The listing builds one solid part. Answer for the finished solid, in the listing's coordinates (mm). A direction names the side the tool comes from. Coordinates: 2 decimals unless noted, no trailing zeros. Order: outer loops, then holes, each group sorted by start corner. A loop starts at its lowest first (then second) coordinate and runs counter-clockwise, first axis right, second up.
Autodesk Inventor part; units mm, degrees
ref_plane "Start Plane" through (0, 0, 25) normal (0, 0, 1) x (1, 0, 0)
ref_plane "End Plane" through (0, 0, 185) normal (0, 0, 1) x (1, 0, 0)
ref_plane "Work Plane4" through (1045, -21, 185) normal (0, 0, 1) x (1, 0, 0)
ref_plane "Start Plane" through (0, 0, 25) normal (0, 0, 1) x (1, 0, 0)
ref_plane "End Plane" through (0, 0, 185) normal (0, 0, 1) x (1, 0, 0)
sketch "Sketch" plane through (0, 0, 0) normal (0, 0, 1) x (1, 0, 0)
  line L0 (-25, -21) -> (-25, 21)
  line L1 (-21, 25) -> (21, 25)
  line L2 (25, 21) -> (25, -21)
  line L3 (21, -25) -> (-21, -25)
  arc A0 (-25, -21) -> (-21, -25) centre (-21, -21) ccw
  arc A1 (25, 21) -> (21, 25) centre (21, 21) ccw
  arc A2 (-21, 25) -> (-25, 21) centre (-21, 21) ccw
  arc A3 (21, -25) -> (25, -21) centre (21, -21) ccw
  arc A4 (-21, 23) -> (-23, 21) centre (-21, 21) ccw
  line L4 (-21, 23) -> (21, 23)
  arc A5 (23, 21) -> (21, 23) centre (21, 21) ccw
  line L5 (23, 21) -> (23, -21)
  arc A6 (21, -23) -> (23, -21) centre (21, -21) ccw
  line L6 (21, -23) -> (-21, -23)
  arc A7 (-23, -21) -> (-21, -23) centre (-21, -21) ccw
  line L7 (-23, -21) -> (-23, 21)
  line L8 (0, 36.1598) -> (0, -36.1598) construction
  line L9 (-36.1598, 0) -> (36.1598, 0) construction
  dimension "d7" = 4
  dimension "d9" = 50
  dimension "d11" = 50
  dimension "d12" = 2
  dimension "d15" = 25
  dimension "d16" = 25
extrude "Body" add sketch "Sketch" along normal up to surface (160 mm away) from surface at 25
sketch "Sketch3" plane through (0, 0, 0) normal (0, 0, 1) x (1, 0, 0)
  line L0 (0, 0) -> (10, 0)
ref_plane "Work Plane3" through (0, 0, 0) normal (0, -1, 0) x (1, 0, 0)
sketch "Sketch4" plane through (0, 0, 0) normal (0, -1, 0) x (1, 0, 0)
  line L0 (-2, 25) -> (12, 25)
  line L1 (-2, 185) -> (12, 185)
  dimension "d18" = 160
ref_plane "Work Plane4" through (1045, -21, 185) normal (0, 0, 1) x (1, 0, 0)
split "Split1" plane through (1045, -21, 185) removes the side toward (0, 0, 1)
ref_plane "Work Plane5" through (-1270, -21, 25) normal (0, 0, -1) x (-1, 0, 0)
split "Split2" plane through (-1270, -21, 25) removes the side toward (0, 0, -1)
equation "\"d7\" = G_IR"
equation "\"d9\" = G_W"
equation "\"d11\" = G_H"
equation "\"d12\" = G_T"
equation "\"d15\" = 0.5 * d9"
equation "\"d16\" = 0.5 * d11"
equation "\"d3\" = G_L"
equation "\"G_W\" = 50"
equation "\"G_H\" = 50"
equation "\"G_T\" = 2"
equation "\"G_IR\" = 4"
equation "\"G_L\" = d18"
equation "\"G_OFFSET_START\" = -25"
equation "\"G_OFFSET_END\" = -25"
equation "\"d13\" = -G_OFFSET_START"
equation "\"d14\" = G_OFFSET_END + B_L"
properties part number "ISO 10799-2 - 50x50x2 - 160" material "Steel, Galvanized"
(1) The mould has two halves that part along X. Classify faces 3 (the flat face through (-23, 0, 104)), 4 (the flat face through (-25, 0, 104)), 5 (the flat face through (25, 0, 104)): pulls with the +X half, pulls with the -X half, needs draft (parallel to the pull), parting line crosses it, or undercut.
(2) A tool of negligible diameter and unlimited length cuts with its end or side. For faces 1 (the cylindrical face through (-23.797, -23.859, 103.88)), 2 (the flat face through (0, -23, 104)), from which of +Z, -Z, +X, -X, +Y, -Y can it reach the whole face along a straight path? Write none if from no direction.
(3) Find section A-A on z = 131. Determine the outline of the cut face in (x, y).
(4) Find the intervals of material crossed by probe 1 along X at (y, z) = (20, 39.5); probe 2 along X at (y, z) = (-22, 79), in increasing order.
(5) Find section B-B on y = -3. Determine the outline of the cut face in (x, z).
Resolved:
1. face 3: undercut
1. face 4: pulls with the -X half
1. face 5: pulls with the +X half
2. face 1: +Z, -Z, -X, -Y
2. face 2: +Z, -Z
3. outline: (-25, -21) arc R4 ccw to (-21, -25) - (21, -25) arc R4 ccw to (25, -21) - (25, 21) arc R4 ccw to (21, 25) - (-21, 25) arc R4 ccw to (-25, 21) - close; hole (-23, -21) arc R2 ccw to (-21, -23) - (21, -23) arc R2 ccw to (23, -21) - (23, 21) arc R2 ccw to (21, 23) - (-21, 23) arc R2 ccw to (-23, 21) - close
4. probe 1: x = -25 to -23, 23 to 25
4. probe 2: x = -24.87 to -22.73, 22.73 to 24.87
5. outline: (-25, 25) - (-23, 25) - (-23, 185) - (-25, 185) - close; (23, 25) - (25, 25) - (25, 185) - (23, 185) - close
